Here's how the part is built. I have some questions about the finished solid (model axes, mm). A direction names the side the tool comes from. Coordinates: 2 decimals unless noted, no trailing zeros. Write each loop counter-clockwise with the first axis right and the second up, starting at its lowest first coordinate (ties: lowest second). Pieces come first, ordered by that corner, then holes.
Item 1: If we section it at B-B (x = 0): Please give me the cut outline in (y, z).
Item 2: If we section it at D-D (z = 1.5): Please give me the cut outline in (x, y), then the cut area to 3 significant figures.
Item 3: I'm going to push flat-ended pins straight in: pin 1 Ø3 at (x, z) = (12, -1) entering from -Y; pin 2 Ø1.5 at (x, z) = (0.5, -0.5) entering from +Y; pin 3 Ø2 at (x, y) = (-8, 2.5) entering from +Z. Where does each tip first touch, or does it pass through?
Item 4: We'd pull the mould along Z, two halves only. Please class faces 1 (the face through (8.11, 3.41, -0.03)), 2 (the face through (-5.3, 3.4, 0)), 3 (the face through (3.418, 1.642, 1.417)), 4 (the face through (-9, 2.5, 1)): +Z half, -Z half, draft (parallel to the pull), parting line (faces both ways), or undercut.
Item 5: If we section it at A-A (y = 3.9): Count the separate pieces of the cut face and the enclosed holes in it, then the cut area to 3 significant figures.
Item 6: If I drill on line 1 (X direction, y = 0.5, z = -2.25); line 2 (Z direction, x = 5, y = 4.1); line 3 (X direction, y = 0.85, z = -0.25), over which ranges is the centre line in solid material (lowest first)?
Item 7: For faces 5 (the face through (1, 1.5, -1)), 6 (the face through (8.318, 3.413, -2.493)), which set-ups out of +Z, -Z, +X, -X, +Y, -Y let a thin tool reach every point of the face, with its end or its side?
from build123d import *

# Parameters (mm, degrees)
CROQUIS1_R              = 3.7
SALIENTE_EXTRUIR2_DEPTH = 4.3
CROQUIS2_R              = 2.5
CORTAR_EXTRUIR1_DEPTH   = 1.5
CROQUIS3_R              = 2.5
CORTAR_EXTRUIR2_DEPTH   = 1
CROQUIS4_R              = 1
CORTAR_EXTRUIR3_DEPTH   = 1.8
SALIENTE_EXTRUIR3_DEPTH = 1.8
CROQUIS6_R              = 0.595
CORTAR_EXTRUIR4_DEPTH   = 1.8


with BuildPart() as part:
    # Croquis1 → Saliente-Extruir2 (new body)
    with BuildSketch(Plane(origin=(0, 0, 0), x_dir=(1, 0, 0), z_dir=(0, 1, 0))):
        Circle(CROQUIS1_R)
    extrude(amount=SALIENTE_EXTRUIR2_DEPTH)

    # Croquis2 → Cortar-Extruir1 (cut)
    with BuildSketch(Plane.XZ):
        Circle(CROQUIS2_R)
    extrude(amount=-CORTAR_EXTRUIR1_DEPTH, mode=Mode.SUBTRACT)

    # Croquis3 → Cortar-Extruir2 (cut)
    with BuildSketch(Plane(origin=(0, 4.3, 0), x_dir=(1, 0, 0), z_dir=(0, 1, 0))):
        Circle(CROQUIS3_R)
    extrude(amount=-CORTAR_EXTRUIR2_DEPTH, mode=Mode.SUBTRACT)

    # Croquis4 → Cortar-Extruir3 (cut)
    with BuildSketch(Plane(origin=(0, 3.3, 0), x_dir=(1, 0, 0), z_dir=(0, 1, 0))):
        Circle(CROQUIS4_R)
    extrude(amount=-CORTAR_EXTRUIR3_DEPTH, mode=Mode.SUBTRACT)

    # Croquis5 → Saliente-Extruir3 (add)
    with BuildSketch(Plane(origin=(0, 4.3, 0), x_dir=(1, 0, 0), z_dir=(0, 1, 0))):
        with BuildLine():
            Line((-2.16564, 3.000000565), (-3.120237459, 0))
            Line((-3.120237459, 0), (-2.16564, -3.000000565))
            Line((-2.16564, -3.000000565), (-14.3, -2))
            ThreePointArc((-14.3, -2), (-16.3, 0), (-14.3, 2))
            Line((-14.3, 2), (-2.16564, 3.000000565))
        make_face()
        with BuildLine():
            Line((3.120237459, 0), (2.16564, -3.000000565))
            Line((2.16564, -3.000000565), (14.3, -2))
            ThreePointArc((14.3, -2), (16.3, 0), (14.3, 2))
            Line((14.3, 2), (2.16564, 3.000000565))
            Line((2.16564, 3.000000565), (3.120237459, 0))
        make_face()
    extrude(amount=-SALIENTE_EXTRUIR3_DEPTH)

    # Croquis6 → Cortar-Extruir4 (cut)
    with BuildSketch(Plane(origin=(0, 4.3, 0), x_dir=(1, 0, 0), z_dir=(0, 1, 0))):
        with Locations((-14.705, 0)):
            Circle(CROQUIS6_R)
        with Locations((-12.705, 0)):
            Circle(CROQUIS6_R)
        with Locations((-10.705, 0)):
            Circle(CROQUIS6_R)
        with Locations((-8.705, 0)):
            Circle(CROQUIS6_R)
        with Locations((-6.705, 0)):
            Circle(CROQUIS6_R)
        with Locations((-4.705, 0)):
            Circle(CROQUIS6_R)
        with Locations((14.705, 0)):
            Circle(CROQUIS6_R)
        with Locations((12.705, 0)):
            Circle(CROQUIS6_R)
        with Locations((10.705, 0)):
            Circle(CROQUIS6_R)
        with Locations((8.705, 0)):
            Circle(CROQUIS6_R)
        with Locations((6.705, 0)):
            Circle(CROQUIS6_R)
        with Locations((4.705, 0)):
            Circle(CROQUIS6_R)
    extrude(amount=-CORTAR_EXTRUIR4_DEPTH, mode=Mode.SUBTRACT)


solid = part.part
Answer list:
1. outline: (0, -3.7) - (4.3, -3.7) - (4.3, -2.5) - (3.3, -2.5) - (3.3, -1) - (1.5, -1) - (1.5, -2.5) - (0, -2.5) - close; (0, 2.5) - (1.5, 2.5) - (1.5, 1) - (3.3, 1) - (3.3, 2.5) - (4.3, 2.5) - (4.3, 3.7) - (0, 3.7) - close
2. outline: (-15.62, 2.5) - (-3.38, 2.5) - (-3.38, 0) - (-2, 0) - (-2, 1.5) - (2, 1.5) - (2, 0) - (3.38, 0) - (3.38, 2.5) - (15.62, 2.5) - (15.62, 4.3) - (2, 4.3) - (2, 3.3) - (-2, 3.3) - (-2, 4.3) - (-15.62, 4.3) - close
2. area: 63.2 mm2
3. pin 1: stops at y = 2.5
3. pin 2: stops at y = 3.3
3. pin 3: stops at z = 2.6
4. face 1: undercut
4. face 2: undercut
4. face 3: parting line
4. face 4: draft
5. separate pieces: 1
5. enclosed holes: 13
5. area: 131 mm2
6. line 1: x = -2.94 to -1.09, 1.09 to 2.94
6. line 2: z = -2.77 to -0.52, 0.52 to 2.77
6. line 3: x = -3.69 to -2.49, 2.49 to 3.69
7. face 5: -Y
7. face 6: -Z, +X, +Y, -Y
